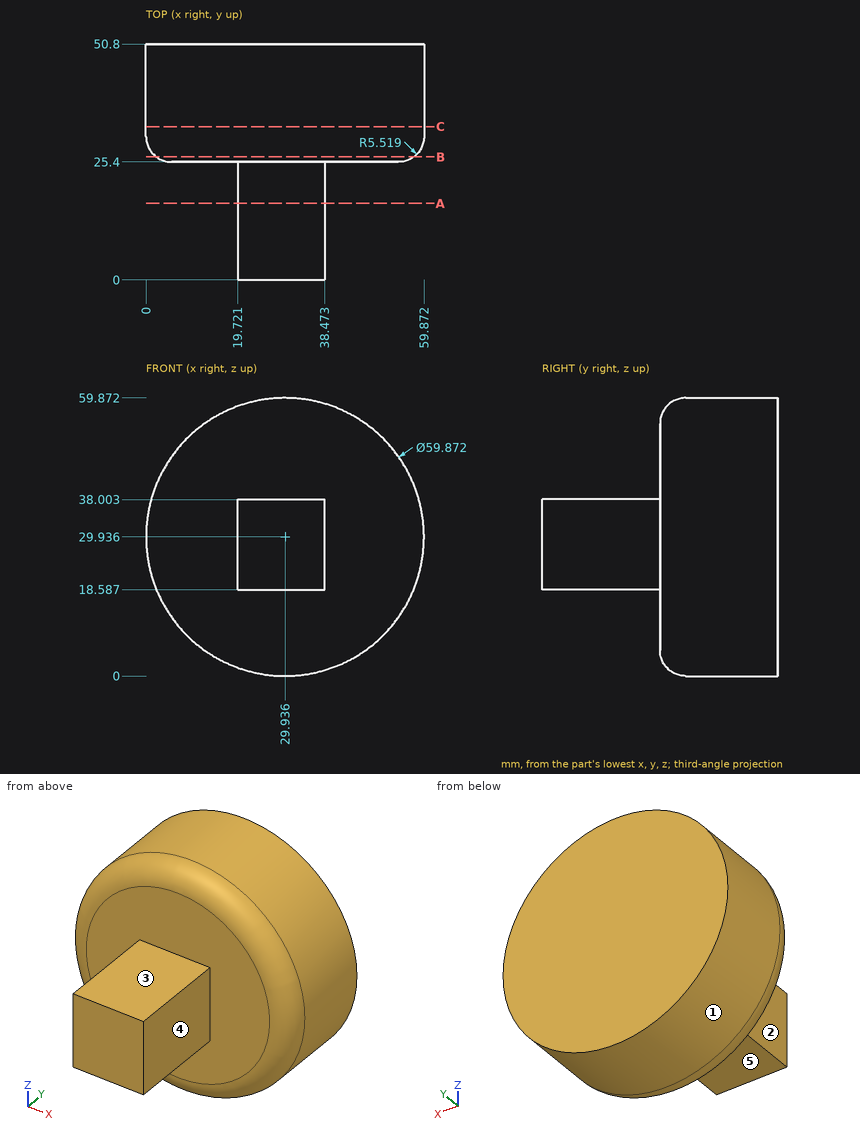
Print and shaded views of the part. All mm, measured from the part's lowest x, y and z. A direction names the side the tool comes from. Coordinates: 2 decimals unless noted, no trailing zeros. Order: outer loops, then holes, each group sorted by start corner. A loop starts at its lowest first (then second) coordinate and runs counter-clockwise, first axis right, second up.
(1) Tool access for the marked faces 1, 2, 3, 4 and 5: list every direction of +Z, -Z, +X, -X, +Y, -Y with a clear straight run to the whole face (end or side of a thin tool).
Check sheet entries:
face 1: +Y, -Y
face 2: +Z, -Z, -X, -Y
face 3: +Z, +X, -X, -Y
face 4: +Z, -Z, +X, -Y
face 5: -Z, +X, -X, -Y
(2) Slice it at A-A, the plane y = 16.5. Write the cut outline in (x, z).
Check sheet entries:
outline: (19.72, 18.59) - (38.47, 18.59) - (38.47, 38) - (19.72, 38) - close
(3) Pin check, flat tips, straight feed: pin 1 Ø20.5 at (x, y) = (27.5, 13.5) entering from -Z; pin 2 Ø4 at (y, z) = (30, 49) entering from -X; pin 3 Ø21.5 at (y, z) = (8, 31.5) entering from +X; pin 4 Ø8 at (x, y) = (45, 21) entering from -Z. Stop position of each tip, or through.
Check sheet entries:
pin 1: stops at z = 18.59
pin 2: stops at x = 5.4
pin 3: stops at x = 38.47
pin 4: passes through
(4) Probe L1, parallel to Z at x = 24.5, y = 21.5; L2, parallel to Y at x = 15.5, z = 44; L3, parallel to X at y = 16, z = 34.5. List the from-to ranges inside material, lowest first.
Check sheet entries:
L1: z = 18.59 to 38
L2: y = 25.4 to 50.8
L3: x = 19.72 to 38.47
(5) Slice it at B-B, the plane y = 26.5. Write the cut outline in (x, z), and give its area (3 significant figures).
Check sheet entries:
outline: circle Ø55.45 at (29.94, 29.94)
area: 2,410 mm2
(6) Slice it at C-C, the plane y = 33. Write the cut outline in (x, z).
Check sheet entries:
outline: circle Ø59.87 at (29.94, 29.94)
